from build123d import *

# Parameters (mm, degrees)
CROQUIS1_W              = 511.5
CROQUIS1_H              = 390
SALIENTE_EXTRUIR1_DEPTH = 2
CROQUIS3_W              = 55
CROQUIS3_H              = 30
CORTAR_EXTRUIR1_DEPTH   = 2
CROQUIS4_W              = 240
CROQUIS4_H              = 125
CORTAR_EXTRUIR2_DEPTH   = 2
CROQUIS5_W              = 40
CROQUIS5_H              = 35
CORTAR_EXTRUIR3_DEPTH   = 2


with BuildPart() as part:
    # Croquis1 → Saliente-Extruir1 (new body)
    with BuildSketch(Plane(origin=(0, 0, 0), x_dir=(1, 0, 0), z_dir=(0, 1, 0))):
        with Locations((255.75, 195)):
            Rectangle(CROQUIS1_W, CROQUIS1_H)
    extrude(amount=SALIENTE_EXTRUIR1_DEPTH)

    # Croquis3 → Cortar-Extruir1 (cut)
    with BuildSketch(Plane(origin=(0, 2, 0), x_dir=(1, 0, 0), z_dir=(0, 1, 0))):
        with Locations((484, 15)):
            Rectangle(CROQUIS3_W, CROQUIS3_H)
        with Locations((27.5, 15)):
            Rectangle(CROQUIS3_W, CROQUIS3_H)
        with Locations((484, 375)):
            Rectangle(CROQUIS3_W, CROQUIS3_H)
        with Locations((27.5, 375)):
            Rectangle(CROQUIS3_W, CROQUIS3_H)
    extrude(amount=-CORTAR_EXTRUIR1_DEPTH, mode=Mode.SUBTRACT)

    # Croquis4 → Cortar-Extruir2 (cut)
    with BuildSketch(Plane(origin=(0, 2, 0), x_dir=(1, 0, 0), z_dir=(0, 1, 0))):
        with Locations((283.5, 62.5)):
            Rectangle(CROQUIS4_W, CROQUIS4_H)
    extrude(amount=-CORTAR_EXTRUIR2_DEPTH, mode=Mode.SUBTRACT)

    # Croquis5 → Cortar-Extruir3 (cut)
    with BuildSketch(Plane(origin=(0, 2, 0), x_dir=(1, 0, 0), z_dir=(0, 1, 0))):
        with Locations((112, 17.5)):
            Rectangle(CROQUIS5_W, CROQUIS5_H)
    extrude(amount=-CORTAR_EXTRUIR3_DEPTH, mode=Mode.SUBTRACT)


solid = part.part
Source: CAD feature listing. Evaluate the final solid. Frame: model axes, mm. Give positions to 0.01 mm unless a question says otherwise; leave off trailing zeros. Write each loop counter-clockwise with the first axis right and the second up, starting at its lowest first coordinate (ties: lowest second). Pieces come first, ordered by that corner, then holes. Notation, with made-up numbers: M -8.75,4 L 10.25,4 A21 ccw 10.25,26 Z; hole C 51,62 d8. An arc over 180 degrees is marked long. Return JSON: item names as keys, results as strings. Group by question number.
1) First-contact query: pin 1 Ø1 at (x, y) = (111.5, 0.5) entering from +Z; pin 2 Ø1 at (x, y) = (267.5, 1) entering from +Z; pin 3 Ø1 at (x, y) = (36, 1) entering from +Z. Flat tips, straight axial feed; report the tip coordinate or a pass-through.
2) Cut plane A-A, the plane z = -105.5. Output: boundary loops of the cut face in (x, y), then the cut area to 3 significant figures.
3) Cut plane B-B, the plane y = 0.7. Output: boundary loops of the cut face in (x, z), then the cut area to 3 significant figures.
4) Ray query, L1, parallel to X at y = 1.25, z = -51.5; L2, parallel to Z at x = 30, y = 0.5; L3, parallel to Z at x = 330, y = 1.6. Return the intervals inside material, ascending.
5) Cut plane D-D, the plane x = 465.5. Output: boundary loops of the cut face in (y, z), then the cut area to 3 significant figures.
6) Cut plane C-C, the plane x = 274.5. Output: boundary loops of the cut face in (y, z), then the cut area to 3 significant figures.
Data:
{
 "1": {"pin 1": "stops at z = -35", "pin 2": "stops at z = -125", "pin 3": "stops at z = -30"},
 "2": {"outline": "M 0,0 L 163.5,0 L 163.5,2 L 0,2 Z; M 403.5,0 L 511.5,0 L 511.5,2 L 403.5,2 Z", "area": "543 mm²"},
 "3": {"outline": "M 0,-360 L 55,-360 L 55,-390 L 456.5,-390 L 456.5,-360 L 511.5,-360 L 511.5,-30 L 456.5,-30 L 456.5,0 L 403.5,0 L 403.5,-125 L 163.5,-125 L 163.5,0 L 132,0 L 132,-35 L 92,-35 L 92,0 L 55,0 L 55,-30 L 0,-30 Z", "area": "161,000 mm²"},
 "4": {"L1": "x = 0 to 163.5, 403.5 to 511.5", "L2": "z = -360 to -30", "L3": "z = -390 to -125"},
 "5": {"outline": "M 0,-360 L 2,-360 L 2,-30 L 0,-30 Z", "area": "660 mm²"},
 "6": {"outline": "M 0,-390 L 2,-390 L 2,-125 L 0,-125 Z", "area": "530 mm²"}
}
